For this review, take the finished solid that the model builds, in its own axes (mm). A direction names the side the tool comes from. Coordinates: 2 decimals unless noted, no trailing zeros. Order: outer loops, then holes, each group sorted by start corner. A loop starts at its lowest first (then second) coordinate and runs counter-clockwise, first axis right, second up. Notation, with made-up numbers: (46, 17.5) -> (71, 17.5) arc R25 cw to (71, 33.5) -> close; hole circle Ø8 at (39.25, 80). An arc over 180 degrees is marked (long way). Write item = value, one per line. Start each with the question number.
1) Consider section B-B on x = 4. Give the boundary of the cut face in (y, z).
2) Wall thickness on probe 1 along X at (y, z) = (36, 3.5); probe 2 along Y at (x, z) = (23, 21.5): over which ranges is each line inside the solid? List them lowest first. Write a range as [from, to].
3) Insertion check: pin 1 Ø12 at (y, z) = (25.5, 8.5) entering from +X; pin 2 Ø10 at (y, z) = (11.5, 4.5) entering from -X; pin 3 Ø12 at (x, y) = (-3.5, 15) entering from -Z. Each pin has a flat end and moves straight along its axis. Give the tip position at first contact, or say it passes through.
4) Machinability: for faces 1 (the face through (20, 24, 10)), 2 (the face through (10, 20, 0)), 3 (the face through (0, 25, 10)), which of the approach directions +Z, -Z, +X, -X, +Y, -Y give a long, thin tool a straight path to every point of the face, cutting with its end or side? Answer none if there is none.
5) Consider section D-D on x = -2.5. Give the boundary of the cut face in (y, z).
6) Consider section C-C on y = 27.5. Give the boundary of the cut face in (x, z), and give its area (3 significant figures).
7) Consider section A-A on z = 18. Give the boundary of the cut face in (x, y), and give its area (3 significant figures).
from build123d import *

# Parameters (mm, degrees)
RESSALTO_EXTRUS_O1_DEPTH = 20
ESBO_O2_W                = 50
ESBO_O2_H                = 50
RESSALTO_EXTRUS_O2_DEPTH = 5


with BuildPart() as part:
    # Esboço1 → Ressalto-extrusão1 (new body)
    with BuildSketch(Plane.XY):
        with BuildLine():
            Line((9, 0), (11, 0))
            ThreePointArc((11, 0), (17.363961031, 2.636038969), (20, 9))
            Line((20, 9), (20, 40))
            Line((20, 40), (0, 40))
            Line((0, 40), (0, 9))
            ThreePointArc((0, 9), (2.636038969, 2.636038969), (9, 0))
        make_face()
    extrude(amount=RESSALTO_EXTRUS_O1_DEPTH)

    # Esboço2 → Ressalto-extrusão2 (add)
    with BuildSketch(Plane(origin=(0, 40, 0), x_dir=(1, 0, 0), z_dir=(0, 1, 0))):
        with Locations((10, -10)):
            Rectangle(ESBO_O2_W, ESBO_O2_H)
    extrude(amount=RESSALTO_EXTRUS_O2_DEPTH)


solid = part.part
Answer sheet:
q1.outline = (1.52, 0) -> (40, 0) -> (40, -15) -> (45, -15) -> (45, 35) -> (40, 35) -> (40, 20) -> (1.52, 20) -> close
q2.probe_1 = [0, 20]
q2.probe_2 = [40, 45]
q3.pin_1 = 20
q3.pin_2 = 0
q3.pin_3 = 0
q4.face_1 = +Z, -Z, +X, -Y
q4.face_2 = -Z, +X, -X, -Y
q4.face_3 = +Z, -Z, -X, -Y
q5.outline = (40, -15) -> (45, -15) -> (45, 35) -> (40, 35) -> close
q6.outline = (0, 0) -> (20, 0) -> (20, 20) -> (0, 20) -> close
q6.area = 400 mm2
q7.outline = (-15, 40) -> (0, 40) -> (0, 9) arc R9 ccw to (9, 0) -> (11, 0) arc R9 ccw to (20, 9) -> (20, 40) -> (35, 40) -> (35, 45) -> (-15, 45) -> close
q7.area = 1,020 mm2
